Part print with two shaded views. Sizes in mm from the minimum x, y, z corner. Round coordinates to 2 decimals unless told otherwise and drop trailing zeros. Order: outer loops, then holes, each group sorted by start corner. A loop starts at its lowest first (then second) coordinate and runs counter-clockwise, first axis right, second up. Notation, with made-up numbers: (89, 72) - (144, 72) arc R25 cw to (144, 108) - close; hole circle Ø2 at (46.25, 48). An arc over 180 degrees is marked (long way). Write item = value, one per line.
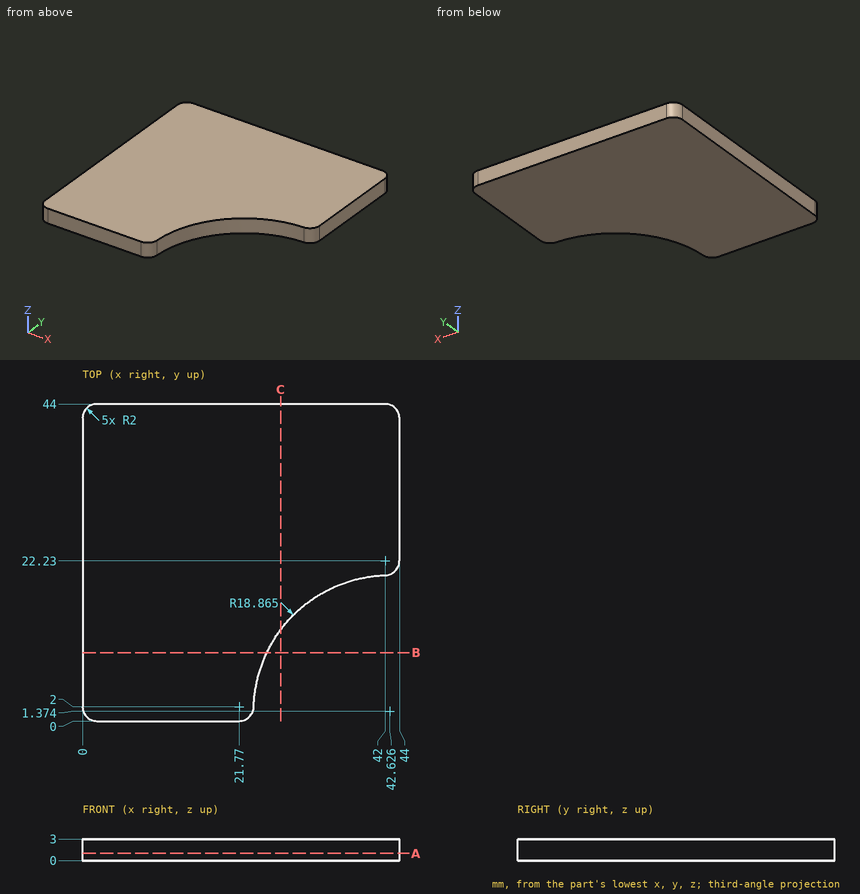
1) Cut at B-B (y = 9.5). Write the cut outline in (x, z), and give its area (3 significant figures).
Conclusion:
outline = (0, 0) - (25.6, 0) - (25.6, 3) - (0, 3) - close
area = 76.8 mm^2
2) Cut at C-C (x = 27.5). Write the cut outline in (y, z).
Conclusion:
outline = (12.65, 0) - (44, 0) - (44, 3) - (12.65, 3) - close
3) Cut at A-A (z = 1). Write the cut outline in (x, y) (1 decimal), and give its area (3 significant figures).
Conclusion:
outline = (0, 2) arc R2 ccw to (2, 0) - (21.8, 0) arc R2 ccw to (23.8, 1.9) arc R18.9 cw to (42.1, 20.2) arc R2 ccw to (44, 22.2) - (44, 42) arc R2 ccw to (42, 44) - (2, 44) arc R2 ccw to (0, 42) - close
area = 1,600 mm^2
4) Wall check: line 1 along Y through (x, z) = (22, 1.5); line 2 along Y through (x, z) = (41, 2.95); line 3 along X through (y, z) = (21, 1.75) (1 decimal). Give the ranges that are in metal, low to high.
Conclusion:
line_1 = 0.01 to 44
line_2 = 20.17 to 44
line_3 = 0 to 43.6
